```python
from build123d import *

# Parameters (mm, degrees)
SKIZZE1_R                       = 22.5
AUFSATZ_LINEAR_AUSTRAGEN1_DEPTH = 2
SKIZZE2_R                       = 19.9
SKIZZE2_R_2                     = 17.9
AUFSATZ_LINEAR_AUSTRAGEN2_DEPTH = 2


with BuildPart() as part:
    # Skizze1 → Aufsatz-Linear austragen1 (new body)
    with BuildSketch(Plane(origin=(0, 0, 0), x_dir=(1, 0, 0), z_dir=(0, 1, 0))):
        with Locations(Location((0, 0, 0), (0, 0, 270))):
            Circle(SKIZZE1_R)
    extrude(amount=AUFSATZ_LINEAR_AUSTRAGEN1_DEPTH)

    # Skizze2 → Aufsatz-Linear austragen2 (add)
    with BuildSketch(Plane(origin=(0, 0, 0), x_dir=(1, 0, 0), z_dir=(0, 1, 0))):
        with Locations(Location((0, 0, 0), (0, 0, 270))):
            Circle(SKIZZE2_R)
        with Locations(Location((0, 0, 0), (0, 0, 270))):
            Circle(SKIZZE2_R_2, mode=Mode.SUBTRACT)
    extrude(amount=-AUFSATZ_LINEAR_AUSTRAGEN2_DEPTH)


solid = part.part
```
Geometry check sheet. Reference: the model listing, model coordinates, mm. A direction names the side the tool comes from. Give positions to 0.01 mm unless a question says otherwise; leave off trailing zeros. Write each loop counter-clockwise with the first axis right and the second up, starting at its lowest first coordinate (ties: lowest second). Pieces come first, ordered by that corner, then holes.
1) Section check C-C, the plane y = -0.8. Record the boundary of the cut face in (x, z), and give its area (3 significant figures).
2) Material ranges on L1, parallel to X at y = -1.1, z = 0; L2, parallel to Y at x = 7, z = 0; L3, parallel to Z at x = -6, y = -0.4, recorded low to high.
3) Section check D-D, the plane z = -18.5. Record the boundary of the cut face in (x, y).
4) Release check for a two-part mould opening along X. For faces 1 (the cylindrical face through (-8.618, 0.986, 20.784)), 2 (the flat face through (0, 2, 0)), 3 (the flat face through (0, 0, 0)) record: pulls with the +X half, pulls with the -X half, needs draft (parallel to the pull), parting line crosses it, or undercut.
5) Section check B-B, the plane x = 0. Record the boundary of the cut face in (y, z).
6) Gauge pin test, flat ends, axial feed: pin 1 (13.5 mm diameter, centred on x = 7, z = -5.5, fed in from -Y); pin 2 (1.5 mm diameter, centred on x = -2, y = 1, fed in from +Z). Record the tip position at first contact, or that the pin passes through.
7) Section check A-A, the plane z = 0. Record the boundary of the cut face in (x, y), and give its area (3 significant figures).
8) Access from +Z, -Z, +X, -X, +Y, -Y to the whole of each face (thin tool, end or side, straight path). Record for faces 4 (the cylindrical face through (-19.427, -0.986, -4.314)), 5 (the flat face through (3, -2, -18)).
Computed:
1. outline: circle Ø39.8 at (0, 0); hole circle Ø35.8 at (0, 0)
1. area: 238 mm2
2. L1: x = -19.9 to -17.9, 17.9 to 19.9
2. L2: y = 0 to 2
2. L3: z = -18.97 to -16.86, 16.86 to 18.97
3. outline: (-12.81, 0) - (-7.33, 0) - (-7.33, -2) - (7.33, -2) - (7.33, 0) - (12.81, 0) - (12.81, 2) - (-12.81, 2) - close
4. face 1: parting line crosses it
4. face 2: needs draft
4. face 3: undercut
5. outline: (-2, -19.9) - (0, -19.9) - (0, -22.5) - (2, -22.5) - (2, 22.5) - (0, 22.5) - (0, 19.9) - (-2, 19.9) - (-2, 17.9) - (0, 17.9) - (0, -17.9) - (-2, -17.9) - close
6. pin 1: stops at y = 0
6. pin 2: stops at z = 22.47
7. outline: (-22.5, 0) - (-19.9, 0) - (-19.9, -2) - (-17.9, -2) - (-17.9, 0) - (17.9, 0) - (17.9, -2) - (19.9, -2) - (19.9, 0) - (22.5, 0) - (22.5, 2) - (-22.5, 2) - close
7. area: 98.0 mm2
8. face 4: -Y
8. face 5: +Z, -Z, +X, -X, -Y
